CAD build for the part. Positions are in the model's coordinates, mm. Face numbers are marked on the shaded views. A direction names the side the tool comes from. Give positions to 0.01 mm unless a question says otherwise; leave off trailing zeros. Write each loop counter-clockwise with the first axis right and the second up, starting at its lowest first coordinate (ties: lowest second). Pieces come first, ordered by that corner, then holes. Notation, with made-up numbers: M -9,2 L 34,2 A21 cw 34,39 Z; hole C 79,39.25 d1. An arc over 180 degrees is marked long. One line per question, with ' | ' between items. Start each with the question number.
1. Which spindle directions (+Z, -Z, +X, -X, +Y, -Y) get a long thin tool onto all of the face, cutting with end or side? Do the marked faces 5, 6, 7, 8 and 9. Say none if no direction does.
2. Cut at B-B, the plane y = -34.5. Write the cut outline in (x, z), then the cut area to 3 significant figures.
3. Pull direction X, two halves, no side cores. Call the marked faces 1, 2, 3 and 4: released by +X, released by -X, zero draft, split by the parting line, or undercut.
4. Cut at C-C, the plane x = 34. Write the cut outline in (y, z).
5. Cut at A-A, the plane y = -2.6. Write the cut outline in (x, z), then the cut area to 3 significant figures.
6. Wall check: L1, parallel to X at y = -6, z = -26.5; L2, parallel to Y at x = 26.5, z = 13; L3, parallel to Z at x = 3, y = 95.5. Give the ranges that are in metal, low to high.
7. Flat gauge pins, fed straight in: pin 1 (4 mm diameter, centred on y = 96.5, z = 3.5, fed in from -X); pin 2 (6 mm diameter, centred on y = 2.5, z = -3.5, fed in from -X); pin 3 (10 mm diameter, centred on y = 34.5, z = -6, fed in from -X). Where does each tip first touch, or does it go through?
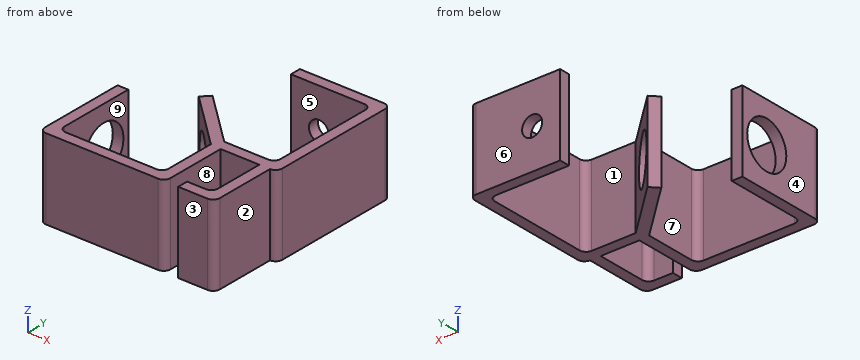
```python
from build123d import *

# Parameters (mm, degrees)
BOSS_EXTRUDE3_DEPTH = 30
SKETCH10_R          = 17.5
CUT_EXTRUDE1_DEPTH  = 8
SKETCH11_R          = 17.5
CUT_EXTRUDE2_DEPTH  = 8
FILLET3_R           = 5
FILLET4_R           = 5
SKETCH12_R          = 7.5
CUT_EXTRUDE3_DEPTH  = 10


with BuildPart() as part:
    # Sketch3 → Boss-Extrude3 (new body, symmetric)
    with BuildSketch(Plane.XY):
        with BuildLine():
            Line((0, 0), (-41.650922989, 38.912730747))
            Line((-41.650922989, 38.912730747), (-36.189487094, 44.758474324))
            Line((-36.189487094, 44.758474324), (4, 7.211102551))
            Line((4, 7.211102551), (37, 7.211102551))
            ThreePointArc((37, 7.211102551), (40.535533906, 8.675568645), (42, 12.211102551))
            Line((42, 12.211102551), (42, 88.211102551))
            ThreePointArc((42, 88.211102551), (40.535533906, 91.746636457), (37, 93.211102551))
            Line((37, 93.211102551), (-18, 93.211102551))
            Line((-18, 93.211102551), (-18, 101.211102551))
            Line((-18, 101.211102551), (45, 101.211102551))
            ThreePointArc((45, 101.211102551), (48.535533906, 99.746636457), (50, 96.211102551))
            Line((50, 96.211102551), (50, 4.211102551))
            ThreePointArc((50, 4.211102551), (48.535533906, 0.675568645), (45, -0.788897449))
            Line((45, -0.788897449), (45, -45.788897449))
            ThreePointArc((45, -45.788897449), (43.535533906, -49.324431355), (40, -50.788897449))
            Line((40, -50.788897449), (18, -50.788897449))
            Line((18, -50.788897449), (18, -42.788897449))
            Line((18, -42.788897449), (32, -42.788897449))
            ThreePointArc((32, -42.788897449), (35.535533906, -41.324431355), (37, -37.788897449))
            Line((37, -37.788897449), (37, -0.788897449))
            Line((37, -0.788897449), (8, -0.788897449))
            Line((8, -0.788897449), (8, -45.788897449))
            ThreePointArc((8, -45.788897449), (6.535533906, -49.324431355), (3, -50.788897449))
            Line((3, -50.788897449), (-86, -50.788897449))
            Line((-86, -50.788897449), (-86, 19.211102551))
            Line((-86, 19.211102551), (-78, 19.211102551))
            Line((-78, 19.211102551), (-78, -42.788897449))
            Line((-78, -42.788897449), (-5, -42.788897449))
            ThreePointArc((-5, -42.788897449), (-1.464466094, -41.324431355), (0, -37.788897449))
            Line((0, -37.788897449), (0, 0))
        make_face()
    extrude(amount=BOSS_EXTRUDE3_DEPTH, both=True)

    # Sketch10 → Cut-Extrude1 (cut)
    with BuildSketch(Plane(origin=(0, 0, 0), x_dir=(0, 0, 1), z_dir=(-0.682679487, -0.730717947, 0))):
        with Locations((0, 35)):
            Circle(SKETCH10_R)
    extrude(amount=-CUT_EXTRUDE1_DEPTH, mode=Mode.SUBTRACT)

    # Sketch11 → Cut-Extrude2 (cut)
    with BuildSketch(Plane.ZY.offset(86)):
        with Locations((0, -2.6)):
            Circle(SKETCH11_R)
    extrude(amount=-CUT_EXTRUDE2_DEPTH, mode=Mode.SUBTRACT)

    # Fillet3
    fillet3_edges = [part.edges().sort_by_distance(p)[0] for p in [
        (-78, -42.788897449, 0),
    ]]
    fillet(fillet3_edges, radius=FILLET3_R)

    # Fillet4
    fillet4_edges = [part.edges().sort_by_distance(p)[0] for p in [
        (-86, -50.788897449, 0),
    ]]
    fillet(fillet4_edges, radius=FILLET4_R)

    # Sketch12 → Cut-Extrude3 (cut)
    with BuildSketch(Plane(origin=(0, 101.211102551, 0), x_dir=(1, 0, 0), z_dir=(0, 1, 0))):
        with Locations((3, 0)):
            Circle(SKETCH12_R)
    extrude(amount=-CUT_EXTRUDE3_DEPTH, mode=Mode.SUBTRACT)


solid = part.part
```
Here are the results:
1) face 5: +Z, -Z, -X | face 6: +Z, -Z, +X, -X, +Y | face 7: +Z, -Z | face 8: +Z, -Z, -Y | face 9: +Z, -Z, +Y
2) outline: M -86,-30 L -78,-30 L -78,30 L -86,30 Z; M 0,-30 L 8,-30 L 8,30 L 0,30 Z; M 37,-30 L 45,-30 L 45,30 L 37,30 Z | area: 1,440 mm^2
3) face 1: undercut | face 2: released by +X | face 3: zero draft | face 4: released by -X
4) outline: M -50.79,-30 L -42.37,-30 L -42.37,30 L -50.79,30 Z; M -0.79,-30 L 7.21,-30 L 7.21,30 L -0.79,30 Z; M 93.21,-30 L 101.21,-30 L 101.21,30 L 93.21,30 Z
5) outline: M -86,-30 L -78,-30 L -78,-17.5 L -86,-17.5 Z; M -86,17.5 L -78,17.5 L -78,30 L -86,30 Z; M 0,-30 L 8,-30 L 8,30 L 0,30 Z; M 37,-30 L 45,-30 L 45,30 L 37,30 Z | area: 1,160 mm^2
6) L1: -86 to -78, 0 to 8, 37 to 45 | L2: -50.79 to -42.79, -0.79 to 7.21, 93.21 to 101.21 | L3: -30 to -7.5, 7.5 to 30
7) pin 1: x = -18 | pin 2: x = -5.89 | pin 3: x = -41.65
